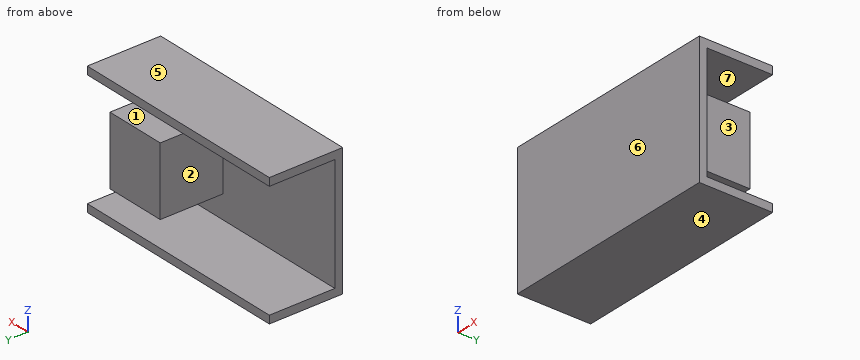
```python
from build123d import *

# Parameters (mm, degrees)
EXTRUDE_1_DEPTH   = 42.5
SKETCH_2_W        = 23.452329067
SKETCH_2_H        = 26.173759744
EXTRUDE_1_2_DEPTH = 24


with BuildPart() as part:
    # 草图1 → Extrude 1 (new, symmetric)
    with BuildSketch(Plane(origin=(0, 0, 0), x_dir=(0, 0, -1), z_dir=(1, 0, 0))):
        Polygon((25, 28), (25, 0), (-25, 0), (-25, 28), (-22, 28), (-22, 3), (22, 3), (22, 28), align=None)
    extrude(amount=EXTRUDE_1_DEPTH, both=True)

    # 草图2 → Extrude 1 2 (add)
    with BuildSketch(Plane(origin=(0, 3, 0), x_dir=(1, 0, 0), z_dir=(0, 1, 0))):
        with Locations((21.393325716, 0)):
            Rectangle(SKETCH_2_W, SKETCH_2_H)
    extrude(amount=EXTRUDE_1_2_DEPTH)


solid = part.part
```
Can you work these out from the model? Positions are in its coordinate system, mm. Face numbers are marked on the shaded views. A direction names the side the tool comes from. Round coordinates to 2 decimals unless told otherwise and drop trailing zeros. Loops run counter-clockwise (first coordinate to the right, second up) from the corner with the lowest first, then second, coordinate; pieces in that order, holes last. Notation, with made-up numbers: M 88.25,-21 L 143.25,-21 A38 ccw 143.25,17 Z; hole C 16,59 d4. An arc over 180 degrees is marked long. Answer as a JSON object with one key per item and string values. Group by question number.
Q1. Will these pins go through, and if not, where does the flat tip stop? pin 1 (12 mm diameter, centred on y = 16.5, z = -13, fed in from +X); pin 2 (4 mm diameter, centred on x = 27.5, z = -17.5, fed in from +Y); pin 3 (10 mm diameter, centred on y = 23.5, z = 0.5, fed in from -X); pin 4 (12 mm diameter, centred on y = 5.5, z = 3, fed in from +X).
Q2. Please list where these lines run through material, in increasing order: L1, parallel to Z at x = 18, y = 16.75; L2, parallel to Z at x = 33.5, y = 17.75; L3, parallel to Y at x = -28, z = -21.5.
Q3. Imagine slicing it at C-C, the plane z = -9. Please give me the cut outline in (x, y).
Q4. Imagine slicing it at B-B, the plane x = 2. Please give me the cut outline in (y, z).
Q5. Imagine slicing it at A-A, the plane y = 14.25. Please give me the cut outline in (x, z), then the cut area to 3 significant figures.
Q6. Imagine slicing it at D-D, the plane x = 22.5. Please give me the cut outline in (y, z).
Q7. We'd pull the mould along Z, two halves only. Please class the marked faces 4, 5, 6 and 7: +Z half, -Z half, draft (parallel to the pull), parting line (faces both ways), or undercut.
Q8. On a 3-axis mill with a long thin cutter (end or side, diameter ignored), from which of +Z, -Z, +X, -X, +Y, -Y can I reach the whole of each face in a straight line? I mean the marked faces 1, 2 and 3. Say none if no direction works.
Findings:
{
 "1": {"pin 1": "stops at x = 33.12", "pin 2": "stops at y = 3", "pin 3": "stops at x = 9.67", "pin 4": "stops at x = 42.5"},
 "2": {"L1": "z = -25 to -22, -13.09 to 13.09, 22 to 25", "L2": "z = -25 to -22, 22 to 25", "L3": "y = 0 to 3"},
 "3": {"outline": "M -42.5,0 L 42.5,0 L 42.5,3 L 33.12,3 L 33.12,27 L 9.67,27 L 9.67,3 L -42.5,3 Z"},
 "4": {"outline": "M 0,-25 L 28,-25 L 28,-22 L 3,-22 L 3,22 L 28,22 L 28,25 L 0,25 Z"},
 "5": {"outline": "M -42.5,-25 L 42.5,-25 L 42.5,-22 L -42.5,-22 Z; M -42.5,22 L 42.5,22 L 42.5,25 L -42.5,25 Z; M 9.67,-13.09 L 33.12,-13.09 L 33.12,13.09 L 9.67,13.09 Z", "area": "1,120 mm2"},
 "6": {"outline": "M 0,-25 L 28,-25 L 28,-22 L 3,-22 L 3,-13.09 L 27,-13.09 L 27,13.09 L 3,13.09 L 3,22 L 28,22 L 28,25 L 0,25 Z"},
 "7": {"face 4": "-Z half", "face 5": "+Z half", "face 6": "draft", "face 7": "undercut"},
 "8": {"face 1": "+X, -X, +Y", "face 2": "-X, +Y", "face 3": "+X, +Y"}
}
